Could you check a few things on this model? Use its own coordinates, in mm. A direction names the side the tool comes from. Give positions to 0.01 mm unless a question says otherwise; leave off trailing zeros. Order: outer loops, then holes, each group sorted by start corner. A loop starts at its lowest first (then second) coordinate and runs counter-clockwise, first axis right, second up. Notation, with made-up numbers: (57.5, 5) -> (62.5, 5) arc R26 ccw to (62.5, 23) -> close; hole circle Ø2 at (-20, 72). An arc over 180 degrees is marked (long way). One line per item, written item: value.
```python
from build123d import *

# Parameters (mm, degrees)
CROQUIS1_R              = 1.5
SALIENTE_EXTRUIR1_DEPTH = 6
CROQUIS2_W              = 2.5
CROQUIS2_H              = 1.5
CORTAR_EXTRUIR1_DEPTH   = 6
REDONDEO3_R             = 1


with BuildPart() as part:
    # Croquis1 → Saliente-Extruir1 (new body)
    with BuildSketch(Plane.XY):
        with BuildLine():
            Line((-3, 0), (-3, -6))
            Line((-3, -6), (3, -6))
            Line((3, -6), (3, 0))
            ThreePointArc((3, 0), (0, 3), (-3, 0))
        make_face()
        Circle(CROQUIS1_R, mode=Mode.SUBTRACT)
    extrude(amount=SALIENTE_EXTRUIR1_DEPTH)

    # Croquis2 → Cortar-Extruir1 (cut, along a direction that is not the sketch's normal)
    with BuildSketch(Plane(origin=(0, 0, 0), x_dir=(-1, 0, 0), z_dir=(0, 0, -1))):
        with Locations((0, -2.75)):
            Rectangle(CROQUIS2_W, CROQUIS2_H)
    extrude(amount=-CORTAR_EXTRUIR1_DEPTH, dir=(0, 0.7071067811865436, -0.7071067811865515), mode=Mode.SUBTRACT)

    # Redondeo3
    redondeo3_edges = [part.edges().sort_by_distance(p)[0] for p in [
        (0, -6, 6),
        (3, -3, 6),
        (0, 3, 6),
        (3, -3, 0),
        (0, -6, 0),
        (-3, -3, 0),
        (0, 3, 0),
        (-3, -3, 6),
        (3, -6, 3),
        (-3, -6, 3),
    ]]
    fillet(redondeo3_edges, radius=REDONDEO3_R)


solid = part.part
```
1) Suppose I cut it at D-D, the plane z = 1.45. Write out the boundary of the cut face in (x, y), then the cut area to 3 significant figures.
Answer below:
outline: (-3, -5) arc R1 ccw to (-2, -6) -> (2, -6) arc R1 ccw to (3, -5) -> (3, 0) arc R3 ccw to (-3, 0) -> close; hole circle Ø3 at (0, 0); hole (-1.25, -4.95) -> (1.25, -4.95) -> (1.25, -3.45) -> (-1.25, -3.45) -> close
area: 38.9 mm2
2) If I drill on line 1 along Z through (x, y) = (0.8, -5); line 2 along Y through (x, z) = (0, 1.55); line 3 along Y through (x, z) = (-0.15, 0.65), over which ranges is the centre line in solid material (lowest first)?
Answer below:
line 1: z = 0 to 1.5, 3 to 6
line 2: y = -6 to -5.05, -3.55 to -1.5, 1.5 to 3
line 3: y = -5.94 to -4.15, -2.65 to -1.49, 1.49 to 2.93
3) Suppose I cut it at A-A, the plane x = 0. Write out the boundary of the cut face in (y, z).
Answer below:
outline: (-6, 1) arc R1 ccw to (-5, 0) -> (-3.5, 0) -> (-6, 2.5) -> close; (-6, 4) -> (-2, 0) -> (-1.5, 0) -> (-1.5, 6) -> (-5, 6) arc R1 ccw to (-6, 5) -> close; (1.5, 0) -> (2, 0) arc R1 ccw to (3, 1) -> (3, 5) arc R1 ccw to (2, 6) -> (1.5, 6) -> close
4) Suppose I cut it at B-B, the plane z = 4.7. Write out the boundary of the cut face in (x, y), then the cut area to 3 significant figures.
Answer below:
outline: (-3, -5) arc R1 ccw to (-2, -6) -> (2, -6) arc R1 ccw to (3, -5) -> (3, 0) arc R3 ccw to (-3, 0) -> close; hole circle Ø3 at (0, 0)
area: 42.6 mm2
5) For faces 1 (the flat face through (0, -4, 2)), 2 (the cylindrical face through (0, 3, 3)), which set-ups out of +Z, -Z, +X, -X, +Y, -Y let a thin tool reach every point of the face, with its end or its side?
Answer below:
face 1: none
face 2: +Z, -Z, +Y
6) Suppose I cut it at C-C, the plane y = -2.5. Write out the boundary of the cut face in (x, z), then the cut area to 3 significant figures.
Answer below:
outline: (-3, 1) arc R1 ccw to (-2, 0) -> (-1.25, 0) -> (-1.25, 0.5) -> (1.25, 0.5) -> (1.25, 0) -> (2, 0) arc R1 ccw to (3, 1) -> (3, 5) arc R1 ccw to (2, 6) -> (-2, 6) arc R1 ccw to (-3, 5) -> close
area: 33.9 mm2
7) We'd pull the mould along Y, two halves only. Please class faces 3 (the cylindrical face through (-2.715, -5.699, 3.028)), 4 (the flat face through (3, -3, 3)), 5 (the flat face through (0, -4.7, 1.2)): +Y half, -Y half, draft (parallel to the pull), parting line (faces both ways), or undercut.
Answer below:
face 3: -Y half
face 4: draft
face 5: undercut
